Can you work these out from the model? Positions are in its coordinate system, mm. A direction names the side the tool comes from. Give positions to 0.01 mm unless a question says otherwise; leave off trailing zeros. Loops run counter-clockwise (first coordinate to the right, second up) from the corner with the lowest first, then second, coordinate; pieces in that order, holes last. Notation, with made-up numbers: (36, -16.5) -> (69, -16.5) arc R27 cw to (69, 0.5) -> close; hole circle Ø9 at (-15, 84). An arc over 180 degrees is marked (long way). Return JSON: item names as keys, results as strings. Group by question number.
Q1. Which directions (+Z, -Z, +X, -X, +Y, -Y) give clear straight access to the entire face, cutting with the end or side of a thin tool? Please do faces 4 (the cylindrical face through (31.39, -19.69, 19.5)), 5 (the flat face through (6.35, 21, 22)), 6 (the flat face through (6.35, 22, -21)), 7 (the flat face through (28, 0, 28.575)), 8 (the cylindrical face through (-0.751, 18.597, 4.13)).
Q2. Suppose I cut it at A-A, the plane z = 0. Please give me the cut outline in (x, y) (3 decimals).
Q3. Thinking about a two-plate mould opening in Z: for faces 1 (the cylindrical face through (31.39, -19.5, -19.69)), 2 (the cylindrical face through (3.131, 25.339, 25.494)), 3 (the flat face through (57.15, 0, 0)), which applies, pulls with the +Z half, pulls with the -Z half, needs draft (parallel to the pull), parting line crosses it, or undercut?
Q4. Will these pins go through, and if not, where does the flat tip stop? pin 1 (14 mm diameter, centred on y = 23.5, z = -22.5, fed in from +X); pin 2 (3 mm diameter, centred on y = 23.622, z = -23.622, fed in from +X); pin 3 (5 mm diameter, centred on y = -6.5, z = -4.5, fed in from -X); pin 4 (6.5 mm diameter, centred on y = -23.622, z = 23.622, fed in from -X).
Q5. I need wall thicknesses on line 1 along X through (y, z) = (0, 21); line 2 along X through (y, z) = (11, -8.5); line 3 along Y through (x, z) = (-10, -1). Which ranges of each line are inside material? Lowest first, please. Write a range as [from, to].
Q6. Suppose I cut it at D-D, the plane x = 5. Please give me the cut outline in (y, z) (3 decimals).
Q7. Suppose I cut it at C-C, the plane x = 23.5. Please give me the cut outline in (y, z) (3 decimals), and give its area (3 significant figures).
```python
from build123d import *

# Parameters (mm, degrees)
SKETCH1_W           = 57.15
SKETCH1_H           = 57.15
SKETCH1_R           = 2.54
BOSS_EXTRUDE1_DEPTH = 6.35
FILLET1_R           = 5.08
SKETCH5_R           = 19.05
BOSS_EXTRUDE4_DEPTH = 1.524
SKETCH6_R           = 3.175
BOSS_EXTRUDE5_DEPTH = 19.05
BOSS_EXTRUDE6_DEPTH = 50.8


with BuildPart() as part:
    # Sketch1 → Boss-Extrude1 (new body)
    with BuildSketch(Plane(origin=(0, 0, 0), x_dir=(0, 0, -1), z_dir=(1, 0, 0))):
        Rectangle(SKETCH1_W, SKETCH1_H)
        with Locations((23.622, 23.622)):
            Circle(SKETCH1_R, mode=Mode.SUBTRACT)
        with Locations((-23.622, 23.622)):
            Circle(SKETCH1_R, mode=Mode.SUBTRACT)
        with Locations((-23.622, -23.622)):
            Circle(SKETCH1_R, mode=Mode.SUBTRACT)
        with Locations((23.622, -23.622)):
            Circle(SKETCH1_R, mode=Mode.SUBTRACT)
    extrude(amount=BOSS_EXTRUDE1_DEPTH)

    # Fillet1
    fillet1_edges = [part.edges().sort_by_distance(p)[0] for p in [
        (3.175, 28.575, 28.575),
        (3.175, 28.575, -28.575),
        (3.175, -28.575, -28.575),
        (3.175, -28.575, 28.575),
    ]]
    fillet(fillet1_edges, radius=FILLET1_R)

    # Sketch5 → Boss-Extrude4 (add)
    with BuildSketch(Plane.ZY):
        with Locations(Location((0, 0, 0), (0, 0, 180))):
            Circle(SKETCH5_R)
    extrude(amount=BOSS_EXTRUDE4_DEPTH)

    # Sketch6 → Boss-Extrude5 (add)
    with BuildSketch(Plane.ZY.offset(1.524)):
        with Locations(Location((0, 0, 0), (0, 0, 180))):
            Circle(SKETCH6_R)
    extrude(amount=BOSS_EXTRUDE5_DEPTH)

    # Sketch7 → Boss-Extrude6 (add)
    with BuildSketch(Plane(origin=(6.35, 0, 0), x_dir=(0, 0, -1), z_dir=(1, 0, 0))):
        with BuildLine():
            Line((-15.875, 28.575), (15.875, 28.575))
            ThreePointArc((15.875, 28.575), (19.594743879, 19.594743879), (28.575, 15.875))
            Line((28.575, 15.875), (28.575, -15.875))
            ThreePointArc((28.575, -15.875), (19.594743879, -19.594743879), (15.875, -28.575))
            Line((15.875, -28.575), (-15.875, -28.575))
            ThreePointArc((-15.875, -28.575), (-19.594743879, -19.594743879), (-28.575, -15.875))
            Line((-28.575, -15.875), (-28.575, 15.875))
            ThreePointArc((-28.575, 15.875), (-19.594743879, 19.594743879), (-15.875, 28.575))
        make_face()
    extrude(amount=BOSS_EXTRUDE6_DEPTH)


solid = part.part
```
Ans:
{
 "1": {"face 4": "+Z, +X, -Y", "face 5": "+Z, +X, +Y", "face 6": "-Z, +X, +Y", "face 7": "+Z, +X, -X, +Y, -Y", "face 8": "-X"},
 "2": {"outline": "(-20.574, -3.175) -> (-1.524, -3.175) -> (-1.524, -19.05) -> (0, -19.05) -> (0, -28.575) -> (57.15, -28.575) -> (57.15, 28.575) -> (0, 28.575) -> (0, 19.05) -> (-1.524, 19.05) -> (-1.524, 3.175) -> (-20.574, 3.175) -> close"},
 "3": {"face 1": "pulls with the -Z half", "face 2": "undercut", "face 3": "needs draft"},
 "4": {"pin 1": "stops at x = 57.15", "pin 2": "passes through", "pin 3": "stops at x = -1.52", "pin 4": "stops at x = 0"},
 "5": {"line 1": "x = [0, 57.15]", "line 2": "x = [-1.52, 57.15]", "line 3": "y = [-3.01, 3.01]"},
 "6": {"outline": "(-28.575, -23.495) arc R5.08 ccw to (-23.495, -28.575) -> (23.495, -28.575) arc R5.08 ccw to (28.575, -23.495) -> (28.575, 23.495) arc R5.08 ccw to (23.495, 28.575) -> (-23.495, 28.575) arc R5.08 ccw to (-28.575, 23.495) -> close; hole circle Ø5.08 at (-23.622, -23.622); hole circle Ø5.08 at (-23.622, 23.622); hole circle Ø5.08 at (23.622, -23.622); hole circle Ø5.08 at (23.622, 23.622)"},
 "7": {"outline": "(-28.575, -15.875) arc R12.7 cw to (-15.875, -28.575) -> (15.875, -28.575) arc R12.7 cw to (28.575, -15.875) -> (28.575, 15.875) arc R12.7 cw to (15.875, 28.575) -> (-15.875, 28.575) arc R12.7 cw to (-28.575, 15.875) -> close", "area": "2,760 mm^2"}
}
